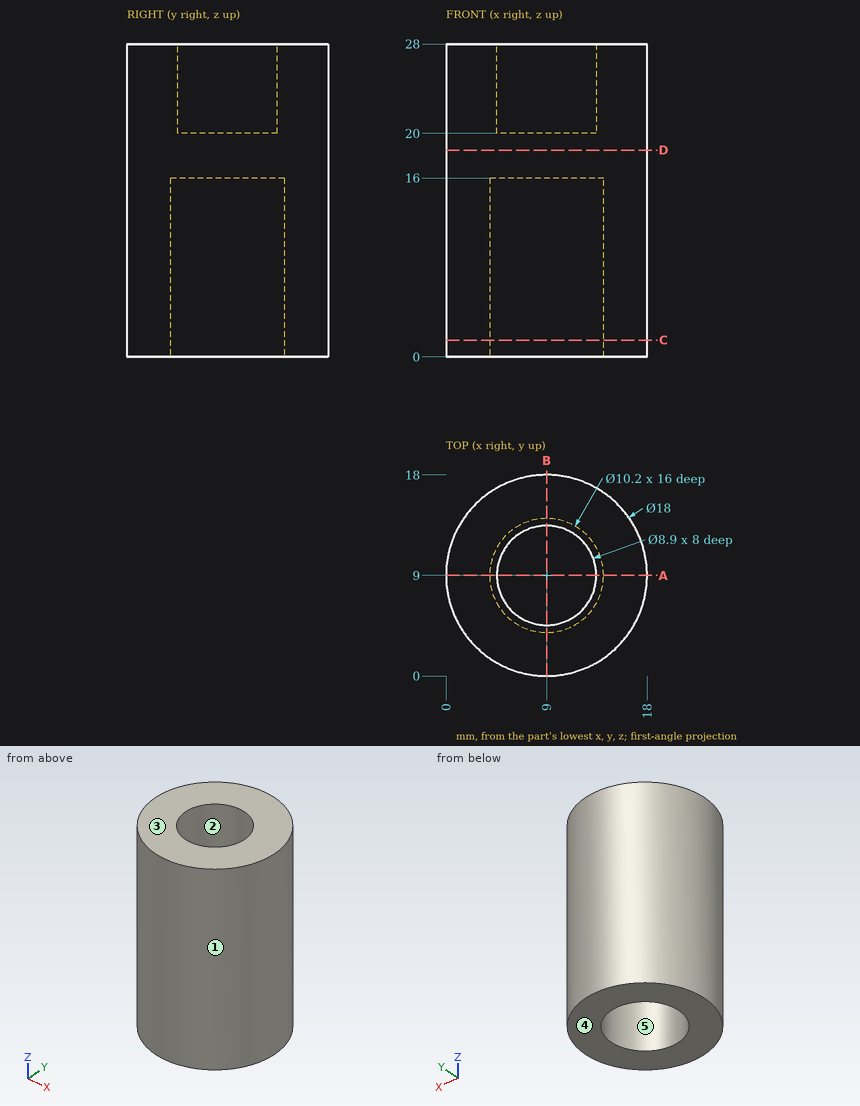
Can you work these out from the drawing? Everything is in mm from the part's minimum corner. A direction names the side the tool comes from. Round coordinates to 2 decimals unless told otherwise and drop trailing zeros. Loops run counter-clockwise (first coordinate to the right, second up) from the corner with the lowest first, then second, coordinate; pieces in that order, holes last. Notation, with made-up numbers: (10, 57) - (55, 57) arc R26 cw to (55, 83) - close; hole circle Ø9 at (-5.75, 49.5). An arc over 180 degrees is marked (long way). Answer in a Markdown table with one row per item. Add a question column.
(1) If we section it at C-C (z = 1.5): Please give me the cut outline in (x, y).
(2) For the marked faces 4 and 5, which set-ups out of +Z, -Z, +X, -X, +Y, -Y let a thin tool reach every point of the face, with its end or its side?
(3) I need wall thicknesses on line 1 along Y through (x, z) = (9, 21.5); line 2 along Y through (x, z) = (9, 3.5); line 3 along Z through (x, y) = (12, 11.5). Which ranges of each line are inside material? Lowest first, please.
(4) If we mould it in two halves opening along Y, with no side actions, what happens to the marked faces 1, 2 and 3? For each: pulls with the +Y half, pulls with the -Y half, needs draft (parallel to the pull), parting line crosses it, or undercut.
(5) If we section it at A-A (y = 9): Please give me the cut outline in (x, z), plus the area to 3 significant figures.
(6) If we section it at D-D (z = 18.5): Please give me the cut outline in (x, y).
(7) I'm going to push flat-ended pins straight in: pin 1 (1.5 mm diameter, centred on x = 12.5, z = 12.5, fed in from +Y); pin 2 (1 mm diameter, centred on y = 2, z = 17.5, fed in from +X); pin 3 (6 mm diameter, centred on x = 15.5, z = 10, fed in from -Y). Where does each tip first touch, or does it pass through?
Model answer:
| question | item | result |
|---|---|---|
| 1 | outline | circle Ø18 at (9, 9); hole circle Ø10.2 at (9, 9) |
| 2 | face 4 | -Z, +X, -X, +Y, -Y |
| 2 | face 5 | -Z |
| 3 | line 1 | y = 0 to 4.55, 13.45 to 18 |
| 3 | line 2 | y = 0 to 3.9, 14.1 to 18 |
| 3 | line 3 | z = 16 to 20 |
| 4 | face 1 | parting line crosses it |
| 4 | face 2 | undercut |
| 4 | face 3 | needs draft |
| 5 | outline | (0, 0) - (3.9, 0) - (3.9, 16) - (14.1, 16) - (14.1, 0) - (18, 0) - (18, 28) - (13.45, 28) - (13.45, 20) - (4.55, 20) - (4.55, 28) - (0, 28) - close |
| 5 | area | 270 mm² |
| 6 | outline | circle Ø18 at (9, 9) |
| 7 | pin 1 | stops at y = 17.57 |
| 7 | pin 2 | stops at x = 15.22 |
| 7 | pin 3 | stops at y = 0.71 |
